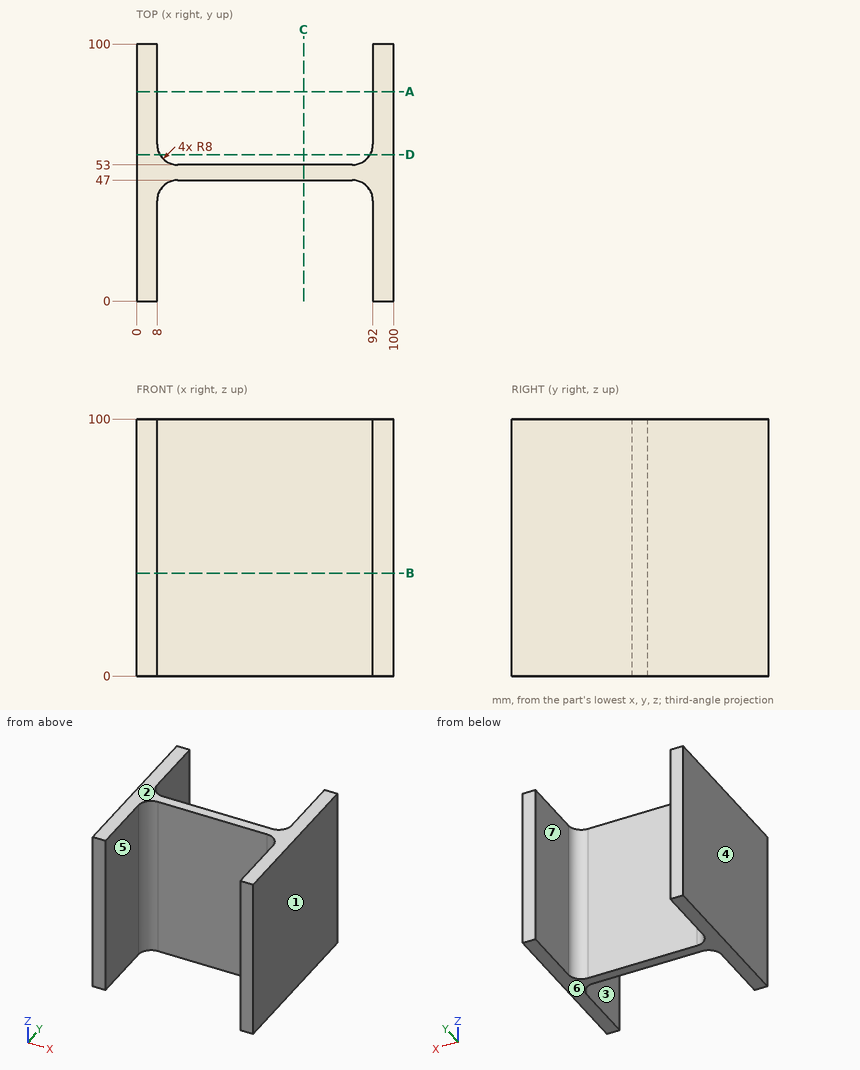
Design review of the part shown in the three views and the two pictorial views. Dimensions are in mm from the part's minimum x, y and z. A direction names the side the tool comes from. Give positions to 0.01 mm unless a question says otherwise; leave off trailing zeros. Write each loop counter-clockwise with the first axis right and the second up, starting at its lowest first coordinate (ties: lowest second). Pieces come first, ordered by that corner, then holes.
(1) Wall thickness on line 1 along X through (y, z) = (37, 21); line 2 along Y through (x, z) = (21.5, 35); line 3 along X through (y, z) = (55.5, 68): over which ranges is each line inside the solid? List them lowest first.
Checked values:
line 1: x = 0 to 8, 92 to 100
line 2: y = 47 to 53
line 3: x = 0 to 10.19, 89.81 to 100
(2) Add section A-A (y = 81.5). Give the boundary of the cut face in (x, z), and give its area (3 significant figures).
Checked values:
outline: (0, 0) - (8, 0) - (8, 100) - (0, 100) - close; (92, 0) - (100, 0) - (100, 100) - (92, 100) - close
area: 1,600 mm2
(3) Clearance check with flat-ended pins moving along their axes: pin 1 Ø3 at (x, z) = (37, 87.5) entering from -Y; pin 2 Ø1.5 at (x, y) = (10.5, 22) entering from +Z; pin 3 Ø1 at (x, z) = (54, 62.5) entering from +Y. State where each tip first meets the part, or that it passes through.
Checked values:
pin 1: stops at y = 47
pin 2: passes through
pin 3: stops at y = 53
(4) Add section D-D (y = 57). Give the boundary of the cut face in (x, z), and give its area (3 significant figures).
Checked values:
outline: (0, 0) - (9.07, 0) - (9.07, 100) - (0, 100) - close; (90.93, 0) - (100, 0) - (100, 100) - (90.93, 100) - close
area: 1,810 mm2
(5) Add section C-C (x = 65). Give the boundary of the cut face in (y, z), and give its area (3 significant figures).
Checked values:
outline: (47, 0) - (53, 0) - (53, 100) - (47, 100) - close
area: 600 mm2
(6) Add section B-B (z = 40). Give the boundary of the cut face in (x, y).
Checked values:
outline: (0, 0) - (8, 0) - (8, 39) arc R8 cw to (16, 47) - (84, 47) arc R8 cw to (92, 39) - (92, 0) - (100, 0) - (100, 100) - (92, 100) - (92, 61) arc R8 cw to (84, 53) - (16, 53) arc R8 cw to (8, 61) - (8, 100) - (0, 100) - close
(7) Tool access review of the marked faces 5, 6 and 7: name each direction out of +Z, -Z, +X, -X, +Y, -Y from which nothing blocks a thin tool from reaching the whole face with its end or side.
Checked values:
face 5: +Z, -Z, -Y
face 6: -Z, +X, -X, +Y, -Y
face 7: +Z, -Z, +Y
(8) Mouldability with a two-part tool opening along X and no side actions: class the marked faces 1, 2, 3 and 4 as +X half, -X half, draft (parallel to the pull), parting line (faces both ways), or undercut.
Checked values:
face 1: +X half
face 2: draft
face 3: undercut
face 4: -X half
